Autodesk Inventor part; units mm, degrees
ref_plane "Work Plane2" through (-74.3, -74.3, -10) normal (0, 0, -1) x (0, 1, 0)
ref_plane "YZ Plane" through (0, 0, 0) normal (1, 0, 0) x (0, 1, 0)
ref_plane "XZ Plane" through (0, 0, 0) normal (0, 1, 0) x (-1, 0, 0)
ref_plane "Work Plane1" through (0, 0, 0) normal (0, 0, 1) x (1, 0, 0)
sketch "Sketch1" plane through (0, 0, 0) normal (0, 0, 1) x (1, 0, 0)
  circle A0 centre (0, 0) radius 62.3
  circle A1 centre (0, 0) radius 49.5
  circle A2 centre (0, 0) radius 61.5
  line L0 (49.5, 0) -> (61.5, 0) construction
  point P0 (55.5, 0)
  point P1 (0, 55.5)
  point P2 (-55.5, 0)
  point P3 (0, -55.5)
  dimension "d0" = 99
  dimension "d1" = 12
  dimension "d4" = 360
ref_plane "Work Plane2" through (-74.3, -74.3, -10) normal (0, 0, -1) x (0, 1, 0)
extrude "Extrusion1" add sketch "Sketch1" against normal up to surface (10 mm away) contours A2
sketch "Sketch2" plane through (0, 0, 0) normal (0, 0, 1) x (1, 0, 0)
  circle A0 centre (0, 0) radius 49.5
  line L0 (49.5, 0) -> (61.5, 0) construction
  circle A1 centre (0, 0) radius 61.5
  point P0 (55.5, 0)
  point P1 (0, 55.5)
  point P2 (-55.5, 0)
  point P3 (0, -55.5)
  dimension "d10" = 360
hole "Hole1" at (55.5, 0, 0) at (0, 55.5, 0) at (-55.5, 0, 0) at (0, -55.5, 0) direction (0, 0, -1) diameter 5 end through all countersink diameter 10.3886 countersink angle 90
properties part number "IR"
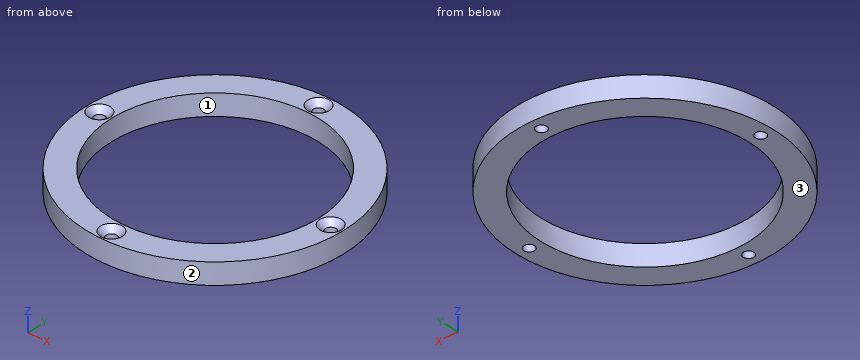
Could you check a few things on this model? Use its own coordinates, in mm. Face numbers are marked on the shaded views. Coordinates: 2 decimals unless noted, no trailing zeros. Loops run counter-clockwise (first coordinate to the right, second up) from the corner with the lowest first, then second, coordinate; pieces in that order, holes last.
1) Thinking about a two-plate mould opening in X: for the marked faces 1, 2 and 3, which applies, released by +X, released by -X, zero draft, split by the parting line, or undercut?
Reported:
face 1: undercut
face 2: split by the parting line
face 3: zero draft
2) Imagine slicing it at C-C (z = -6). List the corners of the cut face in (x, y) for me, and give its area (3 significant figures).
Reported:
outline: circle Ø123 at (0, 0); hole circle Ø5 at (-55.5, 0); hole circle Ø99 at (0, 0); hole circle Ø5 at (0, -55.5); hole circle Ø5 at (0, 55.5); hole circle Ø5 at (55.5, 0)
area: 4,110 mm2
3) Imagine slicing it at A-A (x = 0). List the corners of the cut face in (y, z) for me.
Reported:
outline: (-61.5, -10) - (-58, -10) - (-58, -2.69) - (-60.69, 0) - (-61.5, 0) - close; (-53, -10) - (-49.5, -10) - (-49.5, 0) - (-50.31, 0) - (-53, -2.69) - close; (49.5, -10) - (53, -10) - (53, -2.69) - (50.31, 0) - (49.5, 0) - close; (58, -10) - (61.5, -10) - (61.5, 0) - (60.69, 0) - (58, -2.69) - close
4) Please list where these lines run through material, in increasing order: line 1 along Y through (x, z) = (0, -3.25); line 2 along X through (y, z) = (-1.5, -8.25); line 3 along X through (y, z) = (-4, -5.75).
Reported:
line 1: y = -61.5 to -58, -53 to -49.5, 49.5 to 53, 58 to 61.5
line 2: x = -61.48 to -57.5, -53.5 to -49.48, 49.48 to 53.5, 57.5 to 61.48
line 3: x = -61.37 to -49.34, 49.34 to 61.37
5) Imagine slicing it at D-D (y = -38.5). List the corners of the cut face in (x, z) for me, and give its area (3 significant figures).
Reported:
outline: (-47.96, -10) - (-31.11, -10) - (-31.11, 0) - (-47.96, 0) - close; (31.11, -10) - (47.96, -10) - (47.96, 0) - (31.11, 0) - close
area: 337 mm2
6) Will these pins go through, and if not, where does the flat tip stop? pin 1 Ø5 at (x, z) = (-23, -4) entering from +Y; pin 2 Ø1 at (x, z) = (-44.5, -1.5) entering from -Y; pin 3 Ø2 at (y, z) = (23.5, -6.5) entering from +X.
Reported:
pin 1: stops at y = 57.98
pin 2: stops at y = -42.97
pin 3: stops at x = 57.24
